```python
from build123d import *

# Parameters (mm, degrees)
BOSS_EXTRUDE1_DEPTH = 20


with BuildPart() as part:
    # Sketch2 → Boss-Extrude1 (new body)
    with BuildSketch(Plane(origin=(0, 0, 0), x_dir=(1, 0, 0), z_dir=(0, 1, 0))):
        with BuildLine():
            Line((0, 0), (0, -10))
            ThreePointArc((0, -10), (2.928932188, -17.071067812), (10, -20))
            Line((10, -20), (20, -20))
            Line((20, -20), (20, -30))
            Line((20, -30), (-20, -30))
            Line((-20, -30), (-20, 0))
            Line((-20, 0), (0, 0))
        make_face()
    extrude(amount=BOSS_EXTRUDE1_DEPTH)


with BuildPart() as body_2:
    # Mirror1: mirrored copy
    add(part.part.mirror(Plane(origin=(-20, 20, 30), x_dir=(0, 0, 1), z_dir=(1, 0, 0))))


solid = body_2.part
```
Read the model definition and answer for the solid it produces. Units are mm, in the model's axes. A direction names the side the tool comes from. Round coordinates to 2 decimals unless told otherwise and drop trailing zeros. Write each loop counter-clockwise with the first axis right and the second up, starting at its lowest first coordinate (ties: lowest second). Pieces come first, ordered by that corner, then holes. Notation, with made-up numbers: (29, 75.25) -> (43, 75.25) arc R12 cw to (43, 91.25) -> close; hole circle Ø1 at (55, -10.5). An arc over 180 degrees is marked (long way). Answer in a Markdown table with one row per item. Add a question column.
1) Consider line 1 (Z direction, x = -56, y = 14.75); line 2 (X direction, y = 17.5, z = 9.25); line 3 (Z direction, x = -46, y = 8.25). Determine where each line is inside the solid, lowest interval first.
2) Find section B-B, the plane z = 6. Determine the outline of the cut face in (x, y).
3) Find section C-C, the plane x = -51. Determine the outline of the cut face in (y, z), and give its area (3 significant figures).
4) Find section A-A, the plane y = 16.5. Determine the outline of the cut face in (x, z), and give its area (3 significant figures).
5) Given P1, Ø5, axis at x = -57, y = 14.5, coming from the -Z side; P2, Ø1, axis at y = 17, z = 14, coming from the -X side; P3, Ø8, axis at y = 12, z = 4, coming from the -X side, each flat-ended and moving along its own axis, determine where each tip first touches the part or whether it passes through.
6) Which of the six approach directions +Z, -Z, +X, -X, +Y, -Y give full straight-line access (tool end or side, diameter ignored) to faces 1 (the face through (-20, 10, 15)), 2 (the face through (-40, 10, 5))?
Findings below:
| question | item | result |
|---|---|---|
| 1 | line 1 | 20 to 30 |
| 1 | line 2 | -40 to -20 |
| 1 | line 3 | 19.17 to 30 |
| 2 | outline | (-40, 0) -> (-20, 0) -> (-20, 20) -> (-40, 20) -> close |
| 3 | outline | (0, 20) -> (20, 20) -> (20, 30) -> (0, 30) -> close |
| 3 | area | 200 mm² |
| 4 | outline | (-60, 20) -> (-50, 20) arc R10 cw to (-40, 10) -> (-40, 0) -> (-20, 0) -> (-20, 30) -> (-60, 30) -> close |
| 4 | area | 821 mm² |
| 5 | P1 | z = 20 |
| 5 | P2 | x = -41.07 |
| 5 | P3 | x = -40 |
| 6 | face 1 | +Z, -Z, +X, +Y, -Y |
| 6 | face 2 | -Z, -X, +Y, -Y |
